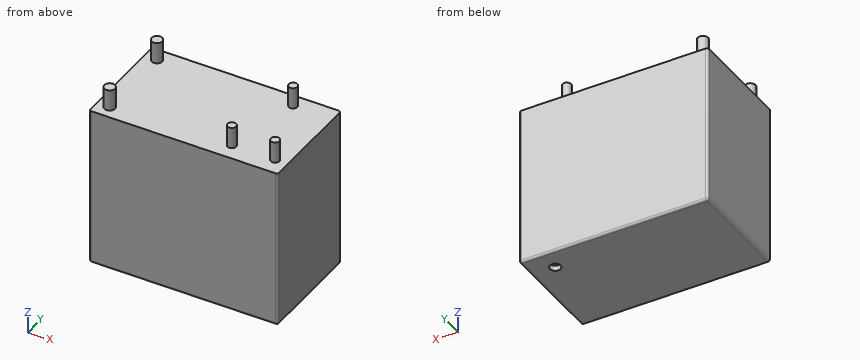
from build123d import *

# Parameters (mm, degrees)
SKETCH_1_W          = 17.6
SKETCH_1_H          = 10.1
EXTRUDE_1_DEPTH     = 15
SKETCH_2_R          = 0.5
SKETCH_2_R_2        = 0.4
EXTRUDE_2_DEPTH     = 2
FILLET_1_R          = 0.2
SKETCH_3_R          = 0.5
CUT_EXTRUDE_1_DEPTH = 0.5


with BuildPart() as part:
    # 草图1 → 凸台-拉伸1 (new body)
    with BuildSketch(Plane.XY):
        with Locations((8.8, 5.05)):
            Rectangle(SKETCH_1_W, SKETCH_1_H)
    extrude(amount=-EXTRUDE_1_DEPTH)

    # 草图2 → 凸台-拉伸2 (add)
    with BuildSketch(Plane.XY):
        with Locations(Location((1.18, 8.85, 0), (0, 0, 180))):
            Circle(SKETCH_2_R)
        with Locations(Location((13.88, 8.85, 0), (0, 0, 180))):
            Circle(SKETCH_2_R_2)
        with Locations(Location((12.38, 1.596982533, 0), (0, 0, 180))):
            Circle(SKETCH_2_R_2)
        with Locations(Location((16.42, 1.596982533, 0), (0, 0, 180))):
            Circle(SKETCH_2_R_2)
        with Locations(Location((1.18, 1.25, 0), (0, 0, 180))):
            Circle(SKETCH_2_R)
    extrude(amount=EXTRUDE_2_DEPTH)

    # 圆角1
    fillet_1_edges = [part.edges().sort_by_distance(p)[0] for p in [
        (17.6, 5.05, -15),
        (8.8, 10.1, -15),
        (0, 5.05, -15),
        (8.8, 0, -15),
        (0, 10.1, -7.5),
        (17.6, 10.1, -7.5),
        (17.6, 0, -7.5),
        (0, 0, -7.5),
    ]]
    fillet(fillet_1_edges, radius=FILLET_1_R)

    # 草图3 → 切除-拉伸1 (cut)
    with BuildSketch(Plane(origin=(0, 0, -15), x_dir=(-1, 0, 0), z_dir=(0, 0, -1))):
        with Locations((-15.4, 8.1)):
            Circle(SKETCH_3_R)
    extrude(amount=-CUT_EXTRUDE_1_DEPTH, mode=Mode.SUBTRACT)


solid = part.part
Geometry: final body of the model. Coordinates: model frame, mm. Coordinates: 2 decimals unless noted, no trailing zeros. Order: outer loops, then holes, each group sorted by start corner. A loop starts at its lowest first (then second) coordinate and runs counter-clockwise, first axis right, second up. Notation, with made-up numbers: (41, 37) - (47, 37) arc R15 cw to (47, 44) - close; hole circle Ø3 at (42, -24.5). An arc over 180 degrees is marked (long way). Use one line per item in the form item = value.
1) Pin query (flat end, axial travel): pin 1 (1 mm diameter, centred on x = 9.5, y = 2.5, fed in from +Z). Return the tip coordinate at first contact, or that it passes through.
Solutions:
pin_1 = 0
2) Section B-B (x = 15.4). Return loops of the section in (y, z), then the cut area to 3 significant figures.
Solutions:
outline = (0, -14.8) arc R0.2 ccw to (0.2, -15) - (7.6, -15) - (7.6, -14.5) - (8.6, -14.5) - (8.6, -15) - (9.9, -15) arc R0.2 ccw to (10.1, -14.8) - (10.1, 0) - (0, 0) - close
area = 151 mm^2
3) Section C-C (y = 4.75). Return loops of the section in (x, z), then the cut area to 3 significant figures.
Solutions:
outline = (0, -14.8) arc R0.2 ccw to (0.2, -15) - (17.4, -15) arc R0.2 ccw to (17.6, -14.8) - (17.6, 0) - (0, 0) - close
area = 264 mm^2
4) Ray query, L1, parallel to Y at x = 15.4, z = -14.75; L2, parallel to Z at x = 6.25, y = 6.5. Return the intervals inside material, ascending.
Solutions:
L1 = 0 to 7.6, 8.6 to 10.1
L2 = -15 to 0
5) Section A-A (y = 8.1). Return loops of the section in (x, z).
Solutions:
outline = (0, -14.8) arc R0.2 ccw to (0.2, -15) - (14.9, -15) - (14.9, -14.5) - (15.9, -14.5) - (15.9, -15) - (17.4, -15) arc R0.2 ccw to (17.6, -14.8) - (17.6, 0) - (0, 0) - close
6) Section D-D (x = 1.18). Return loops of the section in (y, z).
Solutions:
outline = (0, -14.8) arc R0.2 ccw to (0.2, -15) - (9.9, -15) arc R0.2 ccw to (10.1, -14.8) - (10.1, 0) - (9.35, 0) - (9.35, 2) - (8.35, 2) - (8.35, 0) - (1.75, 0) - (1.75, 2) - (0.75, 2) - (0.75, 0) - (0, 0) - close
